Geometry: final body of the model. Coordinates: model frame, mm. Face numbers are marked on the shaded views. A direction names the side the tool comes from. Give positions to 0.01 mm unless a question says otherwise; leave off trailing zeros. Write each loop counter-clockwise with the first axis right and the second up, starting at its lowest first coordinate (ties: lowest second). Pieces come first, ordered by that corner, then holes. Notation, with made-up numbers: M -0.5,71.5 L 53.5,71.5 A19 ccw 53.5,103.5 Z; hole C 34.25,8 d2. An arc over 180 degrees is marked long. Use a Markdown table: item, result. Add a question column.
(1) Draft query along Y for the marked faces 1, 2, 3 and 4. Return one class per face: released by +Y, released by -Y, zero draft, split by the parting line, or undercut.
(2) Material intervals for L1, parallel to Y at x = 46, z = 25; L2, parallel to Y at x = 52.5, z = 5; L3, parallel to Z at x = 51, y = 19.5, sorted ascending.
(3) Reachability of the marked faces 5 and 6 from +Z, -Z, +X, -X, +Y, -Y: full face, straight path, thin tool, end or side. Return the list, or none.
(4) Pin query (flat end, axial travel): pin 1 Ø12 at (y, z) = (35, 25) entering from +X; pin 2 Ø6 at (x, y) = (84, 51.5) entering from -Z. Return the tip coordinate at first contact, or that it passes through.
(5) Cut plane C-C (z = 25). Output: boundary loops of the cut face in (x, y).
(6) Cut plane A-A (y = 35). Output: boundary loops of the cut face in (x, z).
(7) Cut plane D-D (z = 8). Output: boundary loops of the cut face in (x, y).
(8) Cut plane B-B (x = 37). Output: boundary loops of the cut face in (y, z).
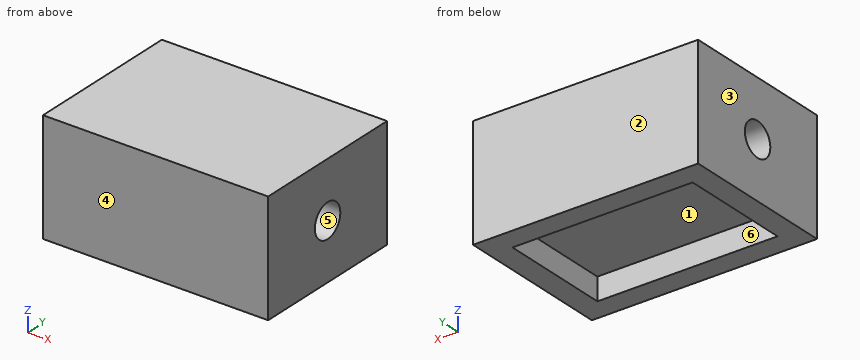
```python
from build123d import *

# Parameters (mm, degrees)
SKETCH1_W           = 100
SKETCH1_H           = 70
BOSS_EXTRUDE1_DEPTH = 50
SKETCH2_R           = 7.5
CUT_EXTRUDE1_DEPTH  = 100
SKETCH3_W           = 80
SKETCH3_H           = 50
CUT_EXTRUDE2_DEPTH  = 10


with BuildPart() as part:
    # Sketch1 → Boss-Extrude1 (new body)
    with BuildSketch(Plane.XY):
        with Locations((50, 35)):
            Rectangle(SKETCH1_W, SKETCH1_H)
    extrude(amount=BOSS_EXTRUDE1_DEPTH)

    # Sketch2 → Cut-Extrude1 (cut)
    with BuildSketch(Plane(origin=(100, 0, 0), x_dir=(0, 0, -1), z_dir=(1, 0, 0))):
        with Locations((-25, 35)):
            Circle(SKETCH2_R)
    extrude(amount=-CUT_EXTRUDE1_DEPTH, mode=Mode.SUBTRACT)

    # Sketch3 → Cut-Extrude2 (cut)
    with BuildSketch(Plane(origin=(0, 0, 0), x_dir=(-1, 0, 0), z_dir=(0, 0, -1))):
        with Locations((-50, 35)):
            Rectangle(SKETCH3_W, SKETCH3_H)
    extrude(amount=-CUT_EXTRUDE2_DEPTH, mode=Mode.SUBTRACT)


solid = part.part
```
Answer list:
| question | item | result |
|---|---|---|
| 1 | face 1 | undercut |
| 1 | face 2 | released by +Y |
| 1 | face 3 | zero draft |
| 1 | face 4 | released by -Y |
| 2 | L1 | 0 to 27.5, 42.5 to 70 |
| 2 | L2 | 0 to 10, 60 to 70 |
| 2 | L3 | 10 to 50 |
| 3 | face 5 | +X, -X |
| 3 | face 6 | -Z |
| 4 | pin 1 | through |
| 4 | pin 2 | z = 10 |
| 5 | outline | M 0,0 L 100,0 L 100,27.5 L 0,27.5 Z; M 0,42.5 L 100,42.5 L 100,70 L 0,70 Z |
| 6 | outline | M 0,0 L 10,0 L 10,10 L 90,10 L 90,0 L 100,0 L 100,17.5 L 0,17.5 Z; M 0,32.5 L 100,32.5 L 100,50 L 0,50 Z |
| 7 | outline | M 0,0 L 100,0 L 100,70 L 0,70 Z; hole M 10,10 L 90,10 L 90,60 L 10,60 Z |
| 8 | outline | M 0,0 L 10,0 L 10,10 L 60,10 L 60,0 L 70,0 L 70,50 L 0,50 Z; hole C 35,25 d15 |
